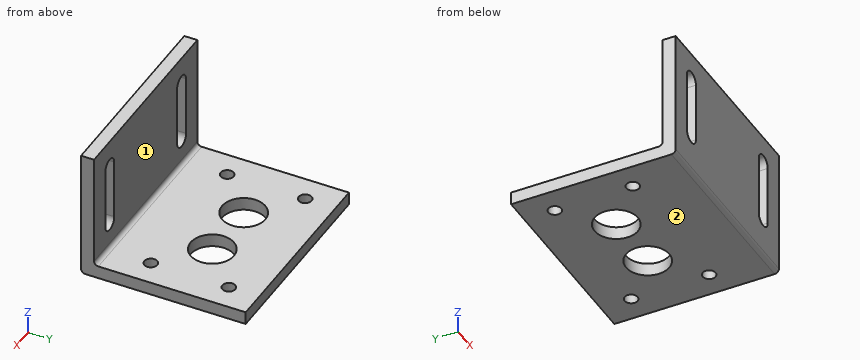
```python
from build123d import *

# Parameters (mm, degrees)
SKETCH_1_W          = 46
SKETCH_1_H          = 30
EXTRUDE_1_DEPTH     = 3
SKETCH_2_W          = 46
SKETCH_2_H          = 38
EXTRUDE_2_DEPTH     = 3
FILLET_1_R          = 1
SKETCH_3_R          = 1.5
SKETCH_3_R_2        = 5
CUT_EXTRUDE_1_DEPTH = 3
CUT_EXTRUDE_2_DEPTH = 3


with BuildPart() as part:
    # 草图1 → 凸台-拉伸1 (new body)
    with BuildSketch(Plane(origin=(0, 0, 0), x_dir=(1, 0, 0), z_dir=(0, 1, 0))):
        Rectangle(SKETCH_1_W, SKETCH_1_H)
    extrude(amount=EXTRUDE_1_DEPTH)

    # 草图2 → 凸台-拉伸2 (add)
    with BuildSketch(Plane(origin=(0, 0, -15), x_dir=(-1, 0, 0), z_dir=(0, 0, -1))):
        with Locations((0, 19)):
            Rectangle(SKETCH_2_W, SKETCH_2_H)
    extrude(amount=-EXTRUDE_2_DEPTH)

    # 圆角1
    fillet_1_edges = [part.edges().sort_by_distance(p)[0] for p in [
        (0, 3, -12),
        (0, 0, -15),
    ]]
    fillet(fillet_1_edges, radius=FILLET_1_R)

    # 草图3 → 切除-拉伸1 (cut)
    with BuildSketch(Plane(origin=(0, 0, -15), x_dir=(-1, 0, 0), z_dir=(0, 0, -1))):
        with Locations((17, 13)):
            Circle(SKETCH_3_R)
        with Locations((17, 31)):
            Circle(SKETCH_3_R)
        with Locations((-17, 31)):
            Circle(SKETCH_3_R)
        with Locations((-17, 13)):
            Circle(SKETCH_3_R)
        with Locations((7, 22)):
            Circle(SKETCH_3_R_2)
        with Locations((-7, 22)):
            Circle(SKETCH_3_R_2)
    extrude(amount=-CUT_EXTRUDE_1_DEPTH, mode=Mode.SUBTRACT)

    # 草图4 → 切除-拉伸2 (cut)
    with BuildSketch(Plane(origin=(0, 3, 0), x_dir=(1, 0, 0), z_dir=(0, 1, 0))):
        with BuildLine():
            Line((-18, -8.4), (-18, 5.6))
            ThreePointArc((-18, 5.6), (-16, 7.6), (-14, 5.6))
            Line((-14, 5.6), (-14, -8.4))
            ThreePointArc((-14, -8.4), (-16, -10.4), (-18, -8.4))
        make_face()
        with BuildLine():
            Line((18, -8.4), (18, 5.6))
            ThreePointArc((18, 5.6), (16, 7.6), (14, 5.6))
            Line((14, 5.6), (14, -8.4))
            ThreePointArc((14, -8.4), (16, -10.4), (18, -8.4))
        make_face()
    extrude(amount=-CUT_EXTRUDE_2_DEPTH, mode=Mode.SUBTRACT)


solid = part.part
```
Verification items for the finished model (mm, model axes). Face numbers are marked on the shaded views. A direction names the side the tool comes from. Round coordinates to 2 decimals unless told otherwise and drop trailing zeros. Write each loop counter-clockwise with the first axis right and the second up, starting at its lowest first coordinate (ties: lowest second). Pieces come first, ordered by that corner, then holes. Notation, with made-up numbers: (20.25, 45.5) -> (37.25, 45.5) arc R6 ccw to (37.25, 56.5) -> close; hole circle Ø5 at (28, 54). An arc over 180 degrees is marked (long way). Write each question's results on one line, items separated by ' | '. Start each with the question number.
1. Cross-section at A-A (y = 31). Enter the section's corners in (x, z), then the cut area to 3 significant figures.
2. Cross-section at B-B (y = 2). Enter the section's corners in (x, z), then the cut area to 3 significant figures.
3. Set-up check for the marked faces 1 and 2: record each of +Z, -Z, +X, -X, +Y, -Y from which the full face is reachable in a straight line by a thin tool's end or side.
4. Material ranges on probe 1 along Y at (x, z) = (17, -13.1); probe 2 along Z at (x, y) = (2.5, 12.5); probe 3 along Y at (x, z) = (7, -12.55), recorded low to high. Write a range as from..to.
5. Cross-section at C-C (z = 3.75). Enter the section's corners in (x, y), then the cut area to 3 significant figures.
6. Cross-section at D-D (x = 17). Enter the section's corners in (y, z).
7. Depth check by flat-ended pin: P1, Ø6, axis at x = -7, y = 22, coming from the -Z side; P2, Ø12, axis at x = -7, z = -2, coming from the +Y side; P3, Ø5, axis at x = 17, y = 31, coming from the +Z side. Enter the tip coordinate at first touch or a pass-through.
Solutions:
1) outline: (-23, -15) -> (-18.5, -15) -> (-18.5, -12) -> (-23, -12) -> close; (-15.5, -15) -> (15.5, -15) -> (15.5, -12) -> (-15.5, -12) -> close; (18.5, -15) -> (23, -15) -> (23, -12) -> (18.5, -12) -> close | area: 120 mm2
2) outline: (-23, -15) -> (23, -15) -> (23, 15) -> (-23, 15) -> close; hole (-18, -5.6) arc R2 ccw to (-14, -5.6) -> (-14, 8.4) arc R2 ccw to (-18, 8.4) -> close; hole (14, -5.6) arc R2 ccw to (18, -5.6) -> (18, 8.4) arc R2 ccw to (14, 8.4) -> close | area: 1,240 mm2
3) face 1: +Z, +X, -X, +Y | face 2: -Z, +X, -X, +Y, -Y
4) probe 1: y = 0..11.5, 14.5..29.5, 32.5..38 | probe 2: z = -15..-12 | probe 3: y = 0..17, 27..38
5) outline: (-23, 0) -> (-18, 0) -> (-18, 3) -> (-23, 3) -> close; (-14, 0) -> (14, 0) -> (14, 3) -> (-14, 3) -> close; (18, 0) -> (23, 0) -> (23, 3) -> (18, 3) -> close | area: 114 mm2
6) outline: (0, -14) arc R1 ccw to (1, -15) -> (11.5, -15) -> (11.5, -12) -> (4, -12) arc R1 cw to (3, -11) -> (3, -7.33) -> (0, -7.33) -> close; (0, 10.13) -> (3, 10.13) -> (3, 15) -> (0, 15) -> close; (14.5, -15) -> (29.5, -15) -> (29.5, -12) -> (14.5, -12) -> close; (32.5, -15) -> (38, -15) -> (38, -12) -> (32.5, -12) -> close
7) P1: passes through | P2: stops at y = 3 | P3: stops at z = -12
